Geometry check sheet. Reference: the model listing, model coordinates, mm. A direction names the side the tool comes from. Give positions to 0.01 mm unless a question says otherwise; leave off trailing zeros. Loops run counter-clockwise (first coordinate to the right, second up) from the corner with the lowest first, then second, coordinate; pieces in that order, holes last.
```python
from build123d import *

# Parameters (mm, degrees)
BOSS_EXTRUDE1_DEPTH                      = 19.05
CBORE_FOR_1_2_HEX_HEAD_BOLT1_D           = 12.7
CBORE_FOR_1_2_HEX_HEAD_BOLT1_DEPTH       = 19.05
CBORE_FOR_1_2_HEX_HEAD_BOLT1_CBORE_D     = 19.05
CBORE_FOR_1_2_HEX_HEAD_BOLT1_CBORE_DEPTH = 8.255
CUT_EXTRUDE1_DEPTH                       = 102.6
SKETCH5_W                                = 40.64
SKETCH5_H                                = 3.175
CUT_EXTRUDE2_DEPTH                       = 140.7
BOSS_EXTRUDE2_DEPTH                      = 76.2


with BuildPart() as part:
    # Sketch1 → Boss-Extrude1 (new body)
    with BuildSketch(Plane(origin=(0, 0, 0), x_dir=(1, 0, 0), z_dir=(0, 1, 0))):
        with BuildLine():
            Line((-54.61, 50.8), (54.61, 50.8))
            ThreePointArc((54.61, 50.8), (65.386307345, 46.336307345), (69.85, 35.56))
            Line((69.85, 35.56), (69.85, -35.56))
            ThreePointArc((69.85, -35.56), (65.386307345, -46.336307345), (54.61, -50.8))
            Line((54.61, -50.8), (-54.61, -50.8))
            ThreePointArc((-54.61, -50.8), (-65.386307345, -46.336307345), (-69.85, -35.56))
            Line((-69.85, -35.56), (-69.85, 35.56))
            ThreePointArc((-69.85, 35.56), (-65.386307345, 46.336307345), (-54.61, 50.8))
        make_face()
    extrude(amount=BOSS_EXTRUDE1_DEPTH)

    # CBORE for 1/2 Hex Head Bolt1
    with Locations(Plane(origin=(0, 19.05, 0), x_dir=(1, 0, 0), z_dir=(0, 1, 0))):
        with Locations((-54.61, 35.56), (54.61, 35.56), (-54.61, -35.56), (54.61, -35.56)):
            CounterBoreHole(CBORE_FOR_1_2_HEX_HEAD_BOLT1_D / 2, CBORE_FOR_1_2_HEX_HEAD_BOLT1_CBORE_D / 2, CBORE_FOR_1_2_HEX_HEAD_BOLT1_CBORE_DEPTH, depth=CBORE_FOR_1_2_HEX_HEAD_BOLT1_DEPTH)

    # Sketch4 → Cut-Extrude1 (cut, through all)
    with BuildSketch(Plane.XY.offset(50.8)):
        with BuildLine():
            Line((-39.37, 0), (-39.37, 6.35))
            Line((-39.37, 6.35), (-6.985, 6.35))
            ThreePointArc((-6.985, 6.35), (0, 13.335), (6.985, 6.35))
            Line((6.985, 6.35), (39.37, 6.35))
            Line((39.37, 6.35), (39.37, 0))
            Line((39.37, 0), (-39.37, 0))
        make_face()
    extrude(amount=-CUT_EXTRUDE1_DEPTH, mode=Mode.SUBTRACT)

    # Sketch5 → Cut-Extrude2 (cut, through all)
    with BuildSketch(Plane.ZY.offset(69.85)):
        with Locations((0, 1.5875)):
            Rectangle(SKETCH5_W, SKETCH5_H)
    extrude(amount=-CUT_EXTRUDE2_DEPTH, mode=Mode.SUBTRACT)

    # Sketch6 → Boss-Extrude2 (add)
    with BuildSketch(Plane(origin=(0, 19.05, 0), x_dir=(1, 0, 0), z_dir=(0, 1, 0))):
        Polygon((-49.53, 6.604), (-34.008673988, -37.075222335), (49.53, -6.669631594), (34.008673988, 37.009590742), align=None)
    extrude(amount=BOSS_EXTRUDE2_DEPTH)


solid = part.part
```
1) Sectioned sample at D-D on z = 1. Enter the section's corners in (x, y) (3 decimals).
2) Sectioned sample at C-C on x = 0. Enter the section's corners in (y, z) (3 decimals).
3) Sectioned sample at B-B on y = 47.5. Enter the section's corners in (x, z).
4) Scan lines: line 1 along X through (y, z) = (5, 35); line 2 along X through (y, z) = (17.25, 35.56) (3 decimals); line 3 along Z through (x, y) = (-54.61, 14) (3 decimals). Record each from-to range of solid material in increasing order.
5) Sectioned sample at A-A on x = 57.5. Enter the section's corners in (y, z) (3 decimals).
6) Tool access check on faces 5 (the cylindrical face through (-60.476, 5.322, -33.128)), 6 (the flat face through (54, 3.175, 0)), 7 (the flat face through (-48, 0, 35)), 8 (the flat face through (39.37, 4, 1)), 9 (the flat face through (61, 10.795, -34)). Record the directions out of +Z, -Z, +X, -X, +Y, -Y that give a thin tool (end or side, any length) a straight path to the whole face; none if there is none.
7) Mould release check, pull along Z, two halves, no side actions. Record for faces 1 (the cylindrical face through (-60.667, 5.322, 33.653)), 2 (the flat face through (-39.37, 4, 1)), 3 (the flat face through (-1, 14, -50.8)), 4 (the flat face through (7.176, 56.617, 22.085)): +Z half, -Z half, draft (parallel to the pull), parting line (faces both ways), or undercut.
8) Depth check by flat-ended pin: P1, Ø1, axis at x = -56, y = 2, coming from the +Z side; P2, Ø3, axis at x = -36, y = 68, coming from the -Z side; P3, Ø5, axis at x = 15.5, z = -15, coming from the -Y side. Enter the tip coordinate at first touch or a pass-through.
Determined:
1. outline: (-69.85, 3.175) - (-39.37, 3.175) - (-39.37, 6.35) - (-6.985, 6.35) arc R6.985 cw to (6.985, 6.35) - (39.37, 6.35) - (39.37, 3.175) - (69.85, 3.175) - (69.85, 19.05) - (47.515, 19.05) - (47.515, 95.25) - (-46.828, 95.25) - (-46.828, 19.05) - (-69.85, 19.05) - close
2. outline: (13.335, -50.8) - (19.05, -50.8) - (19.05, -24.631) - (95.25, -24.631) - (95.25, 24.697) - (19.05, 24.697) - (19.05, 50.8) - (13.335, 50.8) - close
3. outline: (-49.53, -6.6) - (34.01, -37.01) - (49.53, 6.67) - (-34.01, 37.08) - close
4. line 1: x = -69.85 to -60.94, -48.28 to -39.37, 39.37 to 48.28, 60.94 to 69.85
4. line 2: x = -69.85 to -64.135, -45.085 to 45.085, 64.135 to 69.85
4. line 3: z = -50.8 to -45.085, -26.035 to 26.035, 45.085 to 50.8
5. outline: (0, -50.523) - (19.05, -50.523) - (19.05, -44.636) - (10.795, -44.636) - (10.795, -41.214) - (0, -41.214) - close; (0, -29.906) - (10.795, -29.906) - (10.795, -26.484) - (19.05, -26.484) - (19.05, 26.484) - (10.795, 26.484) - (10.795, 29.906) - (0, 29.906) - (0, 20.32) - (3.175, 20.32) - (3.175, -20.32) - (0, -20.32) - close; (0, 41.214) - (10.795, 41.214) - (10.795, 44.636) - (19.05, 44.636) - (19.05, 50.523) - (0, 50.523) - close
6. face 5: +Y, -Y
6. face 6: +X, -X, -Y
6. face 7: +Z, -Z, +X, -X, -Y
6. face 8: +Z, -Z, -Y
6. face 9: +Y
7. face 1: undercut
7. face 2: draft
7. face 3: -Z half
7. face 4: +Z half
8. P1: stops at z = 50.77
8. P2: stops at z = -12.07
8. P3: stops at y = 6.35
